Geometry: see drawing. Coordinates: mm, zero at the bounding-box minimum. A direction names the side the tool comes from. Round coordinates to 2 decimals unless told otherwise and drop trailing zeros. Write each loop counter-clockwise with the first axis right and the second up, starting at its lowest first coordinate (ties: lowest second). Pieces come first, ordered by that corner, then holes.
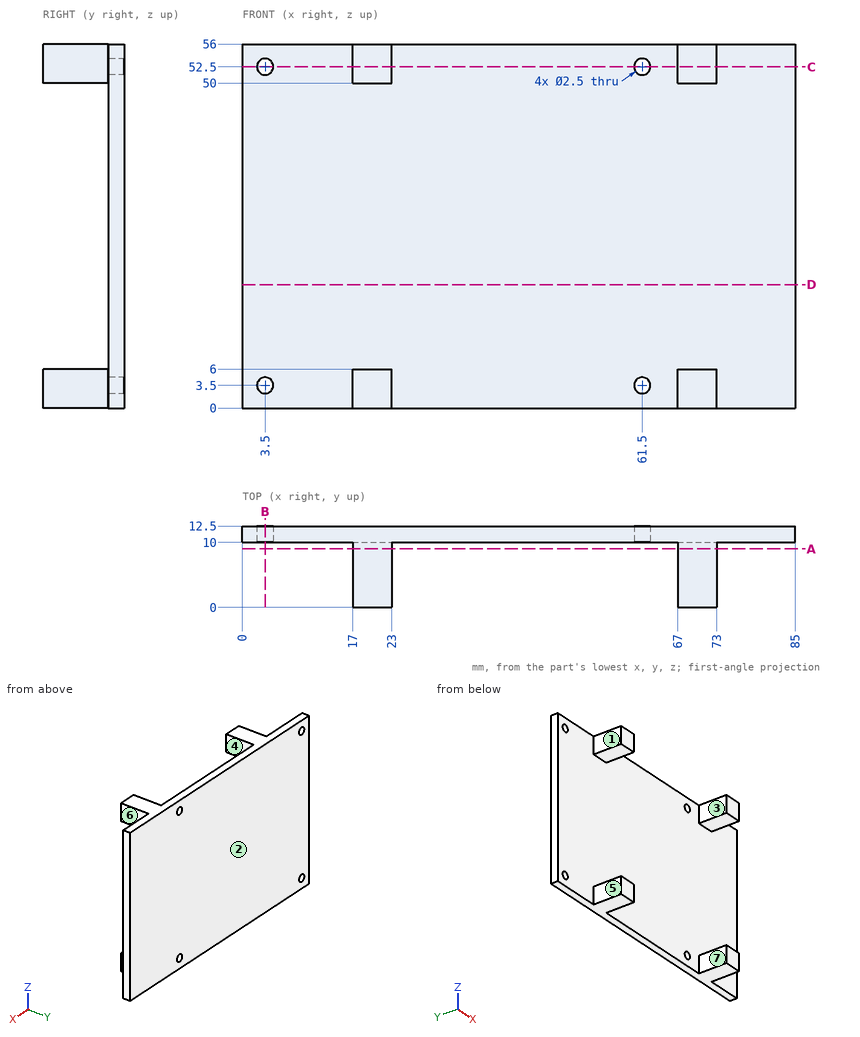
1) Section query B-B on x = 3.5. Return the cut outline in (y, z), then the cut area to 4 significant figures.
Taken from the geometry:
outline: (10, 0) - (12.5, 0) - (12.5, 2.25) - (10, 2.25) - close; (10, 4.75) - (12.5, 4.75) - (12.5, 51.25) - (10, 51.25) - close; (10, 53.75) - (12.5, 53.75) - (12.5, 56) - (10, 56) - close
area: 127.5 mm2
2) Material intervals for line 1 (Z direction, x = 61.5, y = 10.85); line 2 (X direction, y = 9.75, z = 3.5); line 3 (Z direction, x = 68, y = 2.5), sorted ascending.
Taken from the geometry:
line 1: z = 0 to 2.25, 4.75 to 51.25, 53.75 to 56
line 2: x = 17 to 23, 67 to 73
line 3: z = 0 to 6, 50 to 56
3) Section query A-A on y = 9. Return the cut outline in (x, z), then the cut area to 3 significant figures.
Taken from the geometry:
outline: (17, 0) - (23, 0) - (23, 6) - (17, 6) - close; (17, 50) - (23, 50) - (23, 56) - (17, 56) - close; (67, 0) - (73, 0) - (73, 6) - (67, 6) - close; (67, 50) - (73, 50) - (73, 56) - (67, 56) - close
area: 144 mm2
4) Pull-direction query (X, two-part tool) for the marked faces 4, 5, 6 and 7; classes: released by +X, released by -X, zero draft, split by the parting line, or undercut.
Taken from the geometry:
face 4: undercut
face 5: released by -X
face 6: released by +X
face 7: undercut
5) Reachability of the marked faces 1, 2 and 3 from +Z, -Z, +X, -X, +Y, -Y: full face, straight path, thin tool, end or side. Return the list, or none.
Taken from the geometry:
face 1: +Z, -Z, -X, -Y
face 2: +Z, -Z, +X, -X, +Y
face 3: +Z, -Z, -Y
6) Section query D-D on z = 19. Return the cut outline in (x, y).
Taken from the geometry:
outline: (0, 10) - (85, 10) - (85, 12.5) - (0, 12.5) - close
7) Section query C-C on z = 52.5. Return the cut outline in (x, y), then the cut area to 3 significant figures.
Taken from the geometry:
outline: (0, 10) - (2.25, 10) - (2.25, 12.5) - (0, 12.5) - close; (4.75, 10) - (17, 10) - (17, 0) - (23, 0) - (23, 10) - (60.25, 10) - (60.25, 12.5) - (4.75, 12.5) - close; (62.75, 10) - (67, 10) - (67, 0) - (73, 0) - (73, 10) - (85, 10) - (85, 12.5) - (62.75, 12.5) - close
area: 320 mm2
8) Contact query for flat-ended pins moving along their axis: P1, Ø8, axis at x = 51.5, z = 10, coming from the -Y side; P2, Ø3, axis at y = 3.5, z = 54, coming from the -X side; P3, Ø3, axis at y = 3.5, z = 53, coming from the +X side. Output: stop coordinate, or through.
Taken from the geometry:
P1: stops at y = 10
P2: stops at x = 17
P3: stops at x = 73
